Check sheet for the modelled part. Datum: model origin and axes. Units: mm. A direction names the side the tool comes from. Coordinates: 2 decimals unless noted, no trailing zeros. Loops run counter-clockwise (first coordinate to the right, second up) from the corner with the lowest first, then second, coordinate; pieces in that order, holes last. Notation, with made-up numbers: (-19, 35.5) - (32, 35.5) arc R19 cw to (32, 61.5) - close; hole circle Ø1 at (76, 73). An arc over 180 degrees is marked (long way). Write each question's results on one line, items separated by ' | '. Start each with the question number.
1. Cross-section at B-B (y = 7). Record the cut outline in (x, z), and give its area (3 significant figures).
2. Draft check along X on faces 4 (the face through (-20, 15, 1)), 5 (the face through (11.172, -17.146, 1.38)), 6 (the face through (7.515, 23.844, 1.38)), 7 (the face through (0, 0, 0)). Enter one of: released by +X, released by -X, zero draft, split by the parting line, or undercut.
3. Thickness scan on line 1 (Y direction, x = 11, z = 1); line 2 (X direction, y = 19, z = 2.25) (3 decimals); line 3 (X direction, y = -12.5, z = 1.4). Record the ranges inside material, lowest first. Write a range as [from, to].
4. Cross-section at A-A (z = 0.95). Record the cut outline in (x, y) (3 decimals).
5. Cross-section at C-C (x = 0). Record the cut outline in (y, z), and give its area (3 significant figures).
6. Tool access check on faces 1 (the face through (-19.802, -5.165, 1.38)), 2 (the face through (-7.73, -23.775, 1.38)), 3 (the face through (1.375, 20, 1)). Record the directions out of +Z, -Z, +X, -X, +Y, -Y that give a thin tool (end or side, any length) a straight path to the whole face; none if there is none.
7. Gauge pin test, flat ends, axial feed: P1, Ø4, axis at x = 0, y = -12, coming from the -Z side; P2, Ø1.4, axis at y = 22.5, z = 1, coming from the +X side; P3, Ø1.4, axis at y = 21, z = 1, coming from the -X side. Record the tip position at first contact, or that the pin passes through.
```python
from build123d import *

# Parameters (mm, degrees)
CROQUIS1_R              = 25
SALIENTE_EXTRUIR1_DEPTH = 2.8
CROQUIS2_W              = 2.75
CROQUIS2_H              = 18
CORTAR_EXTRUIR1_DEPTH   = 3.8
MATRIZC2_COUNT          = 4
MATRIZC2_ANGLE          = 325.41


with BuildPart() as part:
    # Croquis1 → Saliente-Extruir1 (new body)
    with BuildSketch(Plane.XY):
        Circle(CROQUIS1_R)
    extrude(amount=SALIENTE_EXTRUIR1_DEPTH)

    # Croquis2 → Cortar-Extruir1 (cut, through all)
    with BuildSketch(Plane.XY):
        with Locations((0, 25)):
            Rectangle(CROQUIS2_W, CROQUIS2_H)
    cortar_extruir1 = extrude(amount=CORTAR_EXTRUIR1_DEPTH, mode=Mode.SUBTRACT)

    # MatrizC2: Cortar-Extruir1 ×4 about axis
    matrizc2_axis = Axis((0, 0, 0), (0, 0, 1))
    for i in range(1, MATRIZC2_COUNT):
        add(cortar_extruir1.rotate(matrizc2_axis, i * MATRIZC2_ANGLE / (MATRIZC2_COUNT - 1)), mode=Mode.SUBTRACT)


solid = part.part
```
Established:
1) outline: (-24, 0) - (24, 0) - (24, 2.8) - (-24, 2.8) - close | area: 134 mm^2
2) face 4: released by -X | face 5: undercut | face 6: released by +X | face 7: zero draft
3) line 1: [-22.45, -16.92], [-12.34, 13.53], [18.37, 22.45] | line 2: [-16.248, -1.375], [1.375, 11.432], [14.773, 16.248] | line 3: [-21.65, 10], [11.12, 21.65]
4) outline: (-24.112, -6.604) - (-15.611, -3.765) - (-14.74, -6.373) - (-23.241, -9.212) arc R25 ccw to (13.903, -20.778) - (8.517, -13.615) - (10.715, -11.962) - (16.101, -19.125) arc R25 ccw to (15.303, 19.769) - (10.215, 12.391) - (7.951, 13.952) - (13.039, 21.33) arc R25 ccw to (1.375, 24.962) - (1.375, 16) - (-1.375, 16) - (-1.375, 24.962) arc R25 ccw to start
5) outline: (-25, 0) - (16, 0) - (16, 2.8) - (-25, 2.8) - close | area: 115 mm^2
6) face 1: +Z, -Z | face 2: +Z, -Z, -Y | face 3: +Z, -Z, +Y
7) P1: z = 0 | P2: x = 12.24 | P3: x = -14.59
